Autodesk Inventor part; units mm, degrees
ref_plane "YZ Plane" through (0, 0, 0) normal (1, 0, 0) x (0, 1, 0)
ref_plane "XZ Plane" through (0, 0, 0) normal (0, 1, 0) x (-1, 0, 0)
ref_plane "XY Plane" through (0, 0, 0) normal (0, 0, 1) x (1, 0, 0)
sketch "Esboço1" plane through (0, 0, 0) normal (1, 0, 0) x (0, 1, 0)
  line L0 (0, 0) -> (25, 0)
  line L1 (25, 0) -> (25, -25)
  line L2 (25, -25) -> (0, -25)
  line L3 (0, -25) -> (0, 0)
  dimension "d0" = 25
  dimension "d1" = 25
extrude "Extrusão1" add sketch "Esboço1" along normal blind 2
fillet "Arredondamento1" radius 2 1 edges at (1, 25, 0)
fillet "Arredondamento2" radius 2 1 edges at (1, 0, 0)
fillet "Arredondamento3" radius 2 1 edges at (1, 25, -25)
fillet "Arredondamento4" radius 2 1 edges at (1, 0, -25)
sketch "Esboço2" plane through (2, 0, 0) normal (1, 0, 0) x (0, 0, -1)
  line L0 (23, 25) -> (2, 25)
  line L1 (2, 0) -> (23, 0)
  line L2 (0, 23) -> (0, 2)
  line L3 (0, 12.5) -> (4.75, 12.5)
  line L4 (25, 2) -> (25, 23)
  line L5 (25, 12.5) -> (20.25, 12.5)
  point P0 (0, 0)
  point P1 (12.5, 20.25)
  point P2 (12.5, 4.75)
  dimension "d11" = 4.75
  dimension "d12" = 4.75
hole "Furo1" at (2, 20.25, -12.5) at (2, 4.75, -12.5) direction (-1, 0, 0) diameter 3.242 depth 4 countersink diameter 7.5 countersink angle 90
sketch "Esboço3" plane through (0, 0, 0) normal (-1, 0, 0) x (0, 0, 1)
  line L0 (-25, 2) -> (-25, 23)
  line L1 (-25, 12.5) -> (-20.25, 12.5)
  line L2 (0, 23) -> (0, 2)
  line L3 (0, 12.5) -> (-4.75, 12.5)
  point P0 (0, 0)
  dimension "d20" = 4.75
  dimension "d21" = 4.75
hole "Furo2" at (0, 12.5, -20.25) at (0, 12.5, -4.75) direction (1, 0, 0) diameter 3.242 depth 4 countersink diameter 7.5 countersink angle 90
properties part number "TRILHO FRONTAL"
CAD build for the part. Positions are in the model's coordinates, mm. Round coordinates to 2 decimals unless told otherwise and drop trailing zeros. Order: outer loops, then holes, each group sorted by start corner. A loop starts at its lowest first (then second) coordinate and runs counter-clockwise, first axis right, second up. Notation, with made-up numbers: (-20, -18) -> (4, -18) arc R28 cw to (4, 4) -> close; hole circle Ø2 at (13, 29.5). An arc over 180 degrees is marked (long way). Write item = value, one per line. Start each with the question number.
(1) Cut at A-A, the plane z = -12.5. List the corners of the cut face in (x, y).
(2) Cut at D-D, the plane z = -4.75. List the corners of the cut face in (x, y).
(3) Cut at B-B, the plane x = 0.3. List the corners of the cut face in (y, z), then the cut area to 3 significant figures.
(4) Cut at C-C, the plane y = 20.25. List the corners of the cut face in (x, z).
(5) Probe line 1 (Y direction, x = 1.4, z = -13.25); line 2 (Y direction, x = 0.9, z = -12.5); line 3 (Z direction, x = 1.9, y = 22.5). List the from-to ranges inside material, lowest first. Write a range as [from, to].
Model answer:
q1.outline = (0, 0) -> (2, 0) -> (2, 1) -> (0, 3) -> close; (0, 6.5) -> (2, 8.5) -> (2, 16.5) -> (0, 18.5) -> close; (0, 22) -> (2, 24) -> (2, 25) -> (0, 25) -> close
q2.outline = (0, 0) -> (2, 0) -> (2, 10.75) -> (0, 8.75) -> close; (0, 16.25) -> (2, 14.25) -> (2, 25) -> (0, 25) -> close
q3.outline = (0, -23) arc R2 ccw to (2, -25) -> (23, -25) arc R2 ccw to (25, -23) -> (25, -2) arc R2 ccw to (23, 0) -> (2, 0) arc R2 ccw to (0, -2) -> close; hole circle Ø4.1 at (4.75, -12.5); hole circle Ø6.9 at (12.5, -20.25); hole circle Ø6.9 at (12.5, -4.75); hole circle Ø4.1 at (20.25, -12.5)
q3.area = 520 mm2
q4.outline = (0, -25) -> (2, -25) -> (2, -16.25) -> (0, -14.25) -> close; (0, -10.75) -> (2, -8.75) -> (2, 0) -> (0, 0) -> close
q5.line_1 = [0, 1.69], [7.81, 17.19], [23.31, 25]
q5.line_2 = [0, 2.1], [7.4, 17.6], [22.9, 25]
q5.line_3 = [-25, -15.37], [-9.63, 0]
